Design review of the part built by this model. Coordinates are the model's own, in mm. Give positions to 0.01 mm unless a question says otherwise; leave off trailing zeros. Order: outer loops, then holes, each group sorted by start corner. A loop starts at its lowest first (then second) coordinate and runs counter-clockwise, first axis right, second up. Notation, with made-up numbers: (-7.5, -0.75) -> (26.5, -0.75) arc R13 cw to (26.5, 10.25) -> close; hole circle Ø5 at (44, 43). An arc over 180 degrees is marked (long way). One line per item, written item: value.
Autodesk Fusion 360 part; units mm, degrees
sketch "スケッチ1" plane through (0, 0, 0) normal (0, 1, 0) x (1, 0, 0)
  line L0 (0, 0) -> (74, 0)
  line L1 (74, 0) -> (74, -44)
  line L2 (74, -44) -> (0, -44)
  line L3 (0, -44) -> (0, 0)
  dimension "d1" = 74
  dimension "d2" = 44
extrude "押し出し1" add sketch "スケッチ1" along normal blind 2
sketch "スケッチ2" plane through (0, 0, 0) normal (0, -1, 0) x (1, 0, 0)
  line L0 (74, 44) -> (0, 44)
  line L1 (0, 44) -> (0, 0)
  line L2 (0, 0) -> (74, 0)
  line L3 (74, 0) -> (74, 44)
  line L4 (72, 37) -> (74, 37)
  line L5 (74, 37) -> (74, 31)
  line L6 (74, 31) -> (72, 31)
  line L7 (72, 31) -> (72, 37)
  line L8 (74, 25) -> (74, 19)
  line L9 (74, 19) -> (72, 19)
  line L10 (72, 19) -> (72, 25)
  line L11 (72, 25) -> (74, 25)
  line L12 (74, 13) -> (74, 7)
  line L13 (74, 7) -> (72, 7)
  line L14 (72, 7) -> (72, 13)
  line L15 (72, 13) -> (74, 13)
  line L16 (2, 25) -> (2, 19)
  line L17 (2, 31) -> (0, 31)
  line L18 (2, 37) -> (2, 31)
  line L19 (0, 25) -> (2, 25)
  line L20 (2, 13) -> (2, 7)
  line L21 (0, 19) -> (0, 25)
  line L22 (0, 13) -> (2, 13)
  line L23 (2, 7) -> (0, 7)
  line L24 (0, 31) -> (0, 37)
  line L25 (0, 37) -> (2, 37)
  line L26 (0, 7) -> (0, 13)
  line L27 (2, 19) -> (0, 19)
  line L28 (74, 44) -> (72, 44)
  line L29 (72, 44) -> (72, 42)
  line L30 (72, 42) -> (74, 42)
  line L31 (74, 42) -> (74, 44)
  line L32 (0, 44) -> (2, 44)
  line L33 (2, 44) -> (2, 42)
  line L34 (2, 42) -> (0, 42)
  line L35 (0, 42) -> (0, 44)
  line L36 (0, 0) -> (2, 0)
  line L37 (2, 0) -> (2, 2)
  line L38 (2, 2) -> (0, 2)
  line L39 (0, 2) -> (0, 0)
  line L40 (74, 0) -> (72, 0)
  line L41 (72, 0) -> (72, 2)
  line L42 (72, 2) -> (74, 2)
  line L43 (74, 2) -> (74, 0)
  dimension "d7" = 0
  dimension "d8" = -12
  dimension "d9" = 2
  dimension "d10" = 7
  dimension "d11" = 6
  dimension "d12" = 6
  dimension "d13" = 7
  dimension "d16" = -72
  dimension "d17" = 0
extrude "押し出し2" cut sketch "スケッチ2" against normal blind 2 contours L0 L3 L28 L29 L30 L31 | L0 L1 L32 L33 L34 L35 | L3 L4 L5 L6 L7 | L3 L8 L9 L10 L11 | L1 L17 L18 L24 L25 | L3 L12 L13 L14 L15 | L1 L16 L19 L21 L27 | L2 L3 L40 L41 L42 L43 | L1 L20 L22 L23 L26 | L1 L2 L36 L37 L38 L39
sketch "スケッチ3" plane through (0, 0, 0) normal (0, -1, 0) x (1, 0, 0)
  line L0 (74, 31) -> (72, 31)
  line L1 (72, 31) -> (72, 37)
  line L2 (72, 37) -> (74, 37)
  line L3 (74, 37) -> (74, 42)
  line L4 (74, 42) -> (72, 42)
  line L5 (72, 42) -> (72, 44)
  line L6 (72, 44) -> (2, 44)
  line L7 (2, 44) -> (2, 42)
  line L8 (2, 42) -> (0, 42)
  line L9 (0, 42) -> (0, 37)
  line L10 (0, 37) -> (2, 37)
  line L11 (2, 37) -> (2, 31)
  line L12 (2, 31) -> (0, 31)
  line L13 (0, 31) -> (0, 25)
  line L14 (0, 25) -> (2, 25)
  line L15 (2, 25) -> (2, 19)
  line L16 (2, 19) -> (0, 19)
  line L17 (0, 19) -> (0, 13)
  line L18 (0, 13) -> (2, 13)
  line L19 (2, 13) -> (2, 7)
  line L20 (2, 7) -> (0, 7)
  line L21 (0, 7) -> (0, 2)
  line L22 (0, 2) -> (2, 2)
  line L23 (2, 2) -> (2, 0)
  line L24 (2, 0) -> (72, 0)
  line L25 (72, 0) -> (72, 2)
  line L26 (72, 2) -> (74, 2)
  line L27 (74, 2) -> (74, 7)
  line L28 (74, 7) -> (72, 7)
  line L29 (72, 7) -> (72, 13)
  line L30 (72, 13) -> (74, 13)
  line L31 (74, 13) -> (74, 19)
  line L32 (74, 19) -> (72, 19)
  line L33 (72, 19) -> (72, 25)
  line L34 (72, 25) -> (74, 25)
  line L35 (74, 25) -> (74, 31)
  line L36 (0, 44) -> (7, 44)
  line L37 (7, 44) -> (7, 42)
  line L38 (7, 42) -> (0, 42)
  line L39 (0, 42) -> (0, 44)
  line L40 (16, 42) -> (24, 42)
  line L41 (24, 42) -> (24, 44)
  line L42 (24, 44) -> (16, 44)
  line L43 (16, 44) -> (16, 42)
  line L44 (41, 42) -> (41, 44)
  line L45 (33, 42) -> (41, 42)
  line L46 (41, 44) -> (33, 44)
  line L47 (33, 44) -> (33, 42)
  line L48 (58, 42) -> (58, 44)
  line L49 (50, 42) -> (58, 42)
  line L50 (58, 44) -> (50, 44)
  line L51 (50, 44) -> (50, 42)
  line L52 (67, 42) -> (74, 42)
  line L53 (74, 42) -> (74, 44)
  line L54 (74, 44) -> (67, 44)
  line L55 (67, 44) -> (67, 42)
  line L56 (7, 0) -> (0, 0)
  line L57 (41, 2) -> (33, 2)
  line L58 (33, 2) -> (33, 0)
  line L59 (50, 2) -> (50, 0)
  line L60 (24, 2) -> (16, 2)
  line L61 (24, 0) -> (24, 2)
  line L62 (16, 0) -> (24, 0)
  line L63 (7, 2) -> (7, 0)
  line L64 (50, 0) -> (58, 0)
  line L65 (67, 2) -> (67, 0)
  line L66 (0, 0) -> (0, 2)
  line L67 (74, 2) -> (67, 2)
  line L68 (41, 0) -> (41, 2)
  line L69 (58, 2) -> (50, 2)
  line L70 (16, 2) -> (16, 0)
  line L71 (33, 0) -> (41, 0)
  line L72 (67, 0) -> (74, 0)
  line L73 (58, 0) -> (58, 2)
  line L74 (0, 2) -> (7, 2)
  line L75 (74, 0) -> (74, 2)
  line L76 (72, 0) -> (72, 2)
  line L77 (74, 0) -> (72, 0)
  line L78 (2, 2) -> (2, 0)
  line L79 (2, 0) -> (0, 0)
  dimension "d20" = 8
  dimension "d21" = 2
  dimension "d22" = 2
  dimension "d23" = 9
  dimension "d26" = 17
  dimension "d27" = 0
  dimension "d28" = 2
  dimension "d29" = 9
extrude "押し出し3" cut sketch "スケッチ3" against normal blind 2 contours L4 L5 L52 L53 L54 | L5 L6 L52 L54 L55 | L6 L48 L49 L50 L51 | L25 L26 L67 L72 L75 L76 L77 | L6 L44 L45 L46 L47 | L24 L25 L65 L67 L72 L76 | L6 L40 L41 L42 L43 | L24 L59 L64 L69 L73 | L6 L7 L36 L37 L38 | L7 L8 L36 L38 L39 | L24 L57 L58 L68 L71 | L24 L60 L61 L62 L70 | L23 L24 L56 L63 L74 L78 | L22 L23 L56 L66 L74 L78 L79
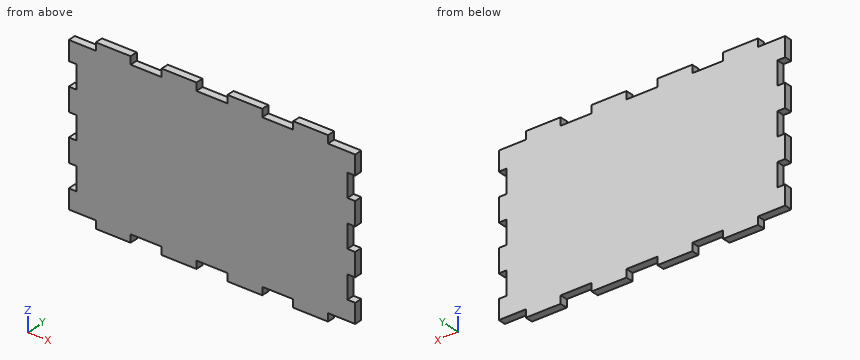
Item 1: Clearance check with flat-ended pins moving along their axes: P1, Ø0.6, axis at x = 1.5, y = 1, coming from the +Z side; P2, Ø0.6, axis at y = 1, z = 43.5, coming from the -X side; P3, Ø1, axis at x = 4, y = 0.5, coming from the -Z side. State where each tip first meets the part, or that it passes through.
Returned:
P1: z = 42
P2: x = 7
P3: z = 2
Item 2: Add section B-B on z = 34.5. Give the boundary of the cut face in (x, y), plus the area to 3 significant figures.
Returned:
outline: (2, 0) -> (72, 0) -> (72, 2) -> (2, 2) -> close
area: 140 mm²
Item 3: To check wall thickness, follow line 1 along X through (y, z) = (1.4, 42.5); line 2 along Z through (x, y) = (16.5, 1.65); line 3 along X through (y, z) = (1.7, 21). State the ranges of each line that lie inside material, in increasing order. Write a range as from..to.
Returned:
line 1: 7..16, 24..33, 41..50, 58..67
line 2: 2..42
line 3: 2..72
Item 4: Add section A-A on x = 68. Give the boundary of the cut face in (y, z).
Returned:
outline: (0, 2) -> (2, 2) -> (2, 42) -> (0, 42) -> close
